```python
from build123d import *

# Parameters (mm, degrees)
F0_R      = 76.2
F1_DEPTH  = 12.7
F2_W      = 19.05
F2_H      = 101.6
F3_DEPTH  = 6.35
F5_DEPTH  = 127.001
F6_W      = 8.89
F6_H      = 30.48
F7_DEPTH  = 33.02
F8_R      = 12.7
F9_R      = 3.556
F10_DEPTH = 95.882075
F11_R     = 3.175
F12_DEPTH = 95.889925


with BuildPart() as f1:
    # F0 (on Top) → F1 (new body)
    with BuildSketch(Plane.XY):
        Circle(F0_R)
    extrude(amount=F1_DEPTH)

    # F2 (on face) → F3 (join)
    with BuildSketch(Plane.XY.offset(12.7)):
        Rectangle(F2_W, F2_H)
    extrude(amount=F3_DEPTH)

    # F4 (on face) → F5 (cut, through all)
    with BuildSketch(Plane.XZ.offset(50.8)):
        Polygon((-3.175, 12.7), (-9.525, 19.05), (-9.525, 12.7), align=None)
        Polygon((9.525, 12.7), (9.525, 19.05), (3.175, 12.7), align=None)
    extrude(amount=-F5_DEPTH, mode=Mode.SUBTRACT)

    # F6 (on face) → F7 (join)
    with BuildSketch(Plane(origin=(0, 0, 0), x_dir=(1, 0, 0), z_dir=(0, 0, -1))):
        with Locations((15.236075, 0)):
            Rectangle(F6_W, F6_H)
        with Locations((-0.003925, 0)):
            Rectangle(F6_W, F6_H)
        with Locations((-15.243925, 0)):
            Rectangle(F6_W, F6_H)
    extrude(amount=F7_DEPTH)

    # F8
    f8_edges = [f1.edges().sort_by_distance(p)[0] for p in [
        (-15.243925, -15.24, -33.02),
        (-15.243925, 15.24, -33.02),
        (-0.003925, -15.24, -33.02),
        (-0.003925, 15.24, -33.02),
        (15.236075, 15.24, -33.02),
        (15.236075, -15.24, -33.02),
    ]]
    fillet(f8_edges, radius=F8_R)

    # F9 (on face) → F10 (cut, through all)
    with BuildSketch(Plane.YZ.offset(19.681075)):
        with Locations((0, -10.823786)):
            Circle(F9_R)
    extrude(amount=-F10_DEPTH, mode=Mode.SUBTRACT)

    # F11 (on face) → F12 (cut, through all)
    with BuildSketch(Plane(origin=(-19.688925, 0, 0), x_dir=(0, -1, 0), z_dir=(-1, 0, 0))):
        with Locations((-8.377785, -21.523021)):
            Circle(F11_R)
        with Locations((0, -24.412786)):
            Circle(F11_R)
        with Locations((8.377784, -21.523022)):
            Circle(F11_R)
    extrude(amount=-F12_DEPTH, mode=Mode.SUBTRACT)


solid = f1.part
```
Work out the finished part from the listing and answer in its coordinate system (mm). A direction names the side the tool comes from. Give positions to 0.01 mm unless a question says otherwise; leave off trailing zeros. Order: outer loops, then holes, each group sorted by start corner. A loop starts at its lowest first (then second) coordinate and runs counter-clockwise, first axis right, second up. Notation, with made-up numbers: (65.5, 22) - (113.5, 22) arc R10 cw to (113.5, 39) - close; hole circle Ø1 at (13.5, -22.75). An arc over 180 degrees is marked (long way). One line per item, written item: value. Start each with the question number.
1. Section C-C, the plane z = 3.5 is taken. Write down the section's boundary in (x, y), then the cut area to 3 significant figures.
2. Section A-A, the plane y = 0 is taken. Count the separate pieces of the cut face and the enclosed holes in it, then the cut area to 3 significant figures.
3. Each of these flat-tipped pins is pushed along its axis until it touches: pin 1 Ø5 at (x, y) = (17, 35.5) entering from -Z; pin 2 Ø2.5 at (x, z) = (-17, -8.5) entering from +Y; pin 3 Ø6 at (x, z) = (34.5, 3) entering from +Y. Where does it stop, or does it pass through?
4. Section D-D, the plane y = -65 is taken. Write down the section's boundary in (x, z), then the cut area to 3 significant figures.
5. Section B-B, the plane x = 0 is taken. Write down the section's boundary in (y, z) (3 decimals).
6. Consider line 1 (X direction, y = 8, z = -3.5); line 2 (Z direction, x = -13.25, y = 0); line 3 (Z direction, x = 0.25, y = 0). Determine where each line is inside the solid, lowest interval first.
7. Which of the six approach directions +Z, -Z, +X, -X, +Y, -Y give full straight-line access (tool end or side, diameter ignored) to faces 5 (the face through (10.791, 0, -16)), 6 (the face through (-60.47, -46.367, 6.261)), 7 (the face through (19.681, 0, -16))?
8. For a pull along Y with two mould halves and no side action, classify faces 1 (the face through (-0.066, -7.964, -18.375)), 2 (the face through (15.174, 6.671, -18.846)), 3 (the face through (16, 1, 12.7)), 4 (the face through (15, -15.24, -10)) as released by +Y, released by -Y, zero draft, split by the parting line, or undercut.
Filled sheet:
1. outline: circle Ø152.4 at (0, 0)
1. area: 18,200 mm²
2. separate pieces: 7
2. enclosed holes: 0
2. area: 2,540 mm²
3. pin 1: z = 0
3. pin 2: y = 15.24
3. pin 3: y = 69.38
4. outline: (-39.77, 0) - (39.77, 0) - (39.77, 12.7) - (-39.77, 12.7) - close
4. area: 1,010 mm²
5. outline: (-76.2, 0) - (-15.24, 0) - (-15.24, -20.32) arc R12.7 ccw to (-2.54, -33.02) - (2.54, -33.02) arc R12.7 ccw to (15.24, -20.32) - (15.24, 0) - (76.2, 0) - (76.2, 12.7) - (50.8, 12.7) - (50.8, 19.05) - (-50.8, 19.05) - (-50.8, 12.7) - (-76.2, 12.7) - close; hole circle Ø6.35 at (-8.378, -21.523); hole circle Ø7.112 at (0, -10.824); hole circle Ø6.35 at (0, -24.413); hole circle Ø6.35 at (8.378, -21.523)
6. line 1: -19.69 to -10.8, -4.45 to 4.44, 10.79 to 19.68
6. line 2: -33.02 to -27.59, -21.24 to -14.38, -7.27 to 12.7
6. line 3: -33.02 to -27.59, -21.24 to -14.38, -7.27 to 19.05
7. face 5: -Z, +Y, -Y
7. face 6: +Z, -Z
7. face 7: -Z, +X, +Y, -Y
8. face 1: undercut
8. face 2: undercut
8. face 3: zero draft
8. face 4: released by -Y
